from build123d import *

# Parameters (mm, degrees)
SKETCH_1_R      = 1.5
SKETCH_1_W      = 8.2
SKETCH_1_H      = 2.2
SKETCH_1_W_2    = 2.2
SKETCH_1_H_2    = 8.2
SKETCH_1_R_2    = 3
EXTRUDE_1_DEPTH = 2


with BuildPart() as part:
    # 草图1 → 凸台-拉伸1 (new body)
    with BuildSketch(Plane.XY):
        Polygon((-68.061769393, -13.095981945), (-52.184883937, -13.095981945), (-18.934883937, -13.095981945), (18.565116063, -13.095981945), (67.695116063, -13.095981945), (171.815116063, 33.779018055), (171.815116063, 73.779018055), (114.815116063, 73.779018055), (114.815116063, 71.279018055), (116.315116063, 71.279018055), (116.315116063, 68.679018055), (114.815116063, 68.679018055), (114.815116063, 65.679018055), (111.815116063, 65.679018055), (111.815116063, 68.679018055), (110.315116063, 68.679018055), (110.315116063, 71.279018055), (111.815116063, 71.279018055), (111.815116063, 73.779018055), (1.315116063, 73.779018055), (1.315116063, 71.279018055), (2.815116063, 71.279018055), (2.815116063, 68.679018055), (1.315116063, 68.679018055), (1.315116063, 65.679018055), (-1.684883937, 65.679018055), (-1.684883937, 68.679018055), (-3.184883937, 68.679018055), (-3.184883937, 71.279018055), (-1.684883937, 71.279018055), (-1.684883937, 73.779018055), (-68.061769393, 73.779018055), (-112.184883937, 73.779018055), (-112.184883937, 71.279018055), (-110.684883937, 71.279018055), (-110.684883937, 68.679018055), (-112.184883937, 68.679018055), (-112.184883937, 65.679018055), (-115.184883937, 65.679018055), (-115.184883937, 68.679018055), (-116.684883937, 68.679018055), (-116.684883937, 71.279018055), (-115.184883937, 71.279018055), (-115.184883937, 73.779018055), (-172.184883937, 73.779018055), (-172.184883937, 33.779018055), align=None)
        with Locations((-33.184883937, -9.095981945)):
            Circle(SKETCH_1_R, mode=Mode.SUBTRACT)
        with Locations((-17.934883937, -9.095981946)):
            Rectangle(SKETCH_1_W, SKETCH_1_H, mode=Mode.SUBTRACT)
        with Locations((-64.184883937, 22.341518055)):
            Rectangle(SKETCH_1_W_2, SKETCH_1_H_2, mode=Mode.SUBTRACT)
        with Locations((17.565116063, -9.095981946)):
            Rectangle(SKETCH_1_W, SKETCH_1_H, mode=Mode.SUBTRACT)
        with Locations((32.815116063, -9.095981945)):
            Circle(SKETCH_1_R, mode=Mode.SUBTRACT)
        with Locations((63.815116063, 22.341518055)):
            Rectangle(SKETCH_1_W_2, SKETCH_1_H_2, mode=Mode.SUBTRACT)
        with BuildLine():
            ThreePointArc((50.815116063, 61.279018055), (52.936436406, 60.400338398), (53.815116063, 58.279018055))
            Line((53.815116063, 58.279018055), (53.815116063, 2.904018055))
            ThreePointArc((53.815116063, 2.904018055), (52.936436406, 0.782697711), (50.815116063, -0.095981945))
            Line((50.815116063, -0.095981945), (-51.184883937, -0.095981945))
            ThreePointArc((-51.184883937, -0.095981945), (-53.306204281, 0.782697711), (-54.184883937, 2.904018055))
            Line((-54.184883937, 2.904018055), (-54.184883937, 58.279018055))
            ThreePointArc((-54.184883937, 58.279018055), (-53.306204281, 60.400338398), (-51.184883937, 61.279018055))
            Line((-51.184883937, 61.279018055), (50.815116063, 61.279018055))
        make_face(mode=Mode.SUBTRACT)
        with Locations((-150.184883937, 53.779018055)):
            Circle(SKETCH_1_R_2, mode=Mode.SUBTRACT)
        Polygon((-140.184883937, 58.879018055), (-125.184883937, 58.879018055), (-102.184883937, 58.879018055), (-102.184883937, 48.679018055), (-125.184883937, 48.679018055), (-140.184883937, 48.679018055), align=None, mode=Mode.SUBTRACT)
        with Locations((-64.184883937, 53.779018055)):
            Circle(SKETCH_1_R, mode=Mode.SUBTRACT)
        with Locations((63.815116063, 53.779018055)):
            Circle(SKETCH_1_R, mode=Mode.SUBTRACT)
        Polygon((139.815116063, 48.679018055), (124.815116063, 48.679018055), (101.815116063, 48.679018055), (101.815116063, 58.879018055), (124.815116063, 58.879018055), (139.815116063, 58.879018055), align=None, mode=Mode.SUBTRACT)
        with Locations((149.815116063, 53.779018055)):
            Circle(SKETCH_1_R_2, mode=Mode.SUBTRACT)
    extrude(amount=EXTRUDE_1_DEPTH)


solid = part.part
Source: CAD feature listing. Evaluate the final solid. Frame: model axes, mm. Give positions to 0.01 mm unless a question says otherwise; leave off trailing zeros. Write each loop counter-clockwise with the first axis right and the second up, starting at its lowest first coordinate (ties: lowest second). Pieces come first, ordered by that corner, then holes. Notation, with made-up numbers: (34.25, 38) -> (90.25, 38) arc R9 cw to (90.25, 43) -> close; hole circle Ø8 at (40, -13). An arc over 180 degrees is marked (long way). Return JSON: item names as keys, results as strings. Group by question number.
1. Section C-C, the plane z = 1.5. Count the separate pieces of the cut face and the enclosed holes in it, then the cut area to 3 significant figures.
2. Section B-B, the plane y = 22.5. Output: boundary loops of the cut face in (x, z), then the cut area to 3 significant figures.
3. Mould query, pull axis X, two halves, no side actions, for faces 1 (the face through (119, 10, 1)), 2 (the face through (-3, -8, 0)), 3 (the face through (-120.85, 10.67, 0.99)), 4 (the face through (-147.323, 54.68, 0.986)). Classes: +X half, -X half, draft (parallel to the pull), parting line (faces both ways), or undercut.
4. Material intervals for line 1 (Y direction, x = 14.5, z = 1.6); line 2 (X direction, y = 57, z = 1.3); line 3 (X direction, y = 44.5, z = 1.05), sorted ascending. Write a range as from..to.
5. Section A-A, the plane x = 37.5. Output: boundary loops of the cut face in (y, z).
6. Section D-D, the plane y = -4. Output: boundary loops of the cut face in (x, z).
7. Pin query (flat end, axial travel): pin 1 Ø1 at (x, y) = (74, -2.5) entering from -Z; pin 2 Ø1 at (y, z) = (24.5, 1) entering from +X. Return the tip coordinate at first contact, or that it passes through.
Determined:
{
 "1": {"separate pieces": "1", "enclosed holes": "13", "area": "17,400 mm2"},
 "2": {"outline": "(-147.13, 0) -> (-65.28, 0) -> (-65.28, 2) -> (-147.13, 2) -> close; (-63.08, 0) -> (-54.18, 0) -> (-54.18, 2) -> (-63.08, 2) -> close; (53.82, 0) -> (62.72, 0) -> (62.72, 2) -> (53.82, 2) -> close; (64.92, 0) -> (146.76, 0) -> (146.76, 2) -> (64.92, 2) -> close", "area": "363 mm2"},
 "3": {"face 1": "+X half", "face 2": "draft", "face 3": "-X half", "face 4": "undercut"},
 "4": {"line 1": "y = -13.1..-10.2, -8..-0.1, 61.28..73.78", "line 2": "x = -172.18..-140.18, -102.18..-54.18, 53.82..101.82, 139.82..171.82", "line 3": "x = -172.18..-54.18, 53.82..171.82"},
 "5": {"outline": "(-13.1, 0) -> (-0.1, 0) -> (-0.1, 2) -> (-13.1, 2) -> close; (61.28, 0) -> (73.78, 0) -> (73.78, 2) -> (61.28, 2) -> close"},
 "6": {"outline": "(-88.27, 0) -> (87.9, 0) -> (87.9, 2) -> (-88.27, 2) -> close"},
 "7": {"pin 1": "stops at z = 0", "pin 2": "stops at x = 152.31"}
}
